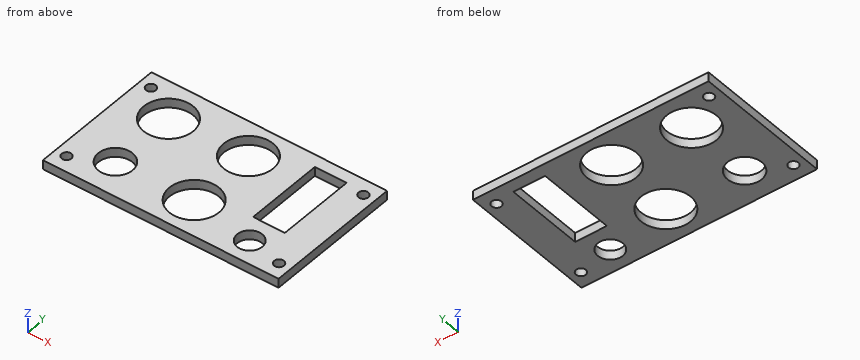
```python
from build123d import *

# Parameters (mm, degrees)
CROQUIS1_W              = 77
CROQUIS1_H              = 45
SALIENTE_EXTRUIR1_DEPTH = 3
CORTAR_EXTRUIR1_REACH   = 5
CROQUIS2_R              = 8.1
CROQUIS2_R_2            = 5.6
CROQUIS2_R_3            = 4.1
CROQUIS2_R_4            = 1.6
CROQUIS2_W              = 10.36
CROQUIS2_H              = 25.6


with BuildPart() as part:
    # Croquis1 → Saliente-Extruir1 (new body)
    with BuildSketch(Plane.XY):
        with Locations((38.5, 22.5)):
            Rectangle(CROQUIS1_W, CROQUIS1_H)
    extrude(amount=SALIENTE_EXTRUIR1_DEPTH)

    # Croquis2 → Cortar-Extruir1 (cut, up to next)
    with BuildSketch(Plane.XY.offset(3), mode=Mode.PRIVATE) as cortar_extruir1_sk1:
        with Locations((15, 33)):
            Circle(CROQUIS2_R)
    cortar_extruir1_tool1 = extrude(cortar_extruir1_sk1.sketch, amount=-CORTAR_EXTRUIR1_REACH, mode=Mode.PRIVATE) & part.part
    add(cortar_extruir1_tool1.solids().sort_by_distance((15, 33, 3))[0], mode=Mode.SUBTRACT)
    # Croquis2 → Cortar-Extruir1 (cut, up to next)
    with BuildSketch(Plane.XY.offset(3), mode=Mode.PRIVATE) as cortar_extruir1_sk2:
        with Locations((15, 11)):
            Circle(CROQUIS2_R_2)
    cortar_extruir1_tool2 = extrude(cortar_extruir1_sk2.sketch, amount=-CORTAR_EXTRUIR1_REACH, mode=Mode.PRIVATE) & part.part
    add(cortar_extruir1_tool2.solids().sort_by_distance((15, 11, 3))[0], mode=Mode.SUBTRACT)
    # Croquis2 → Cortar-Extruir1 (cut, up to next)
    with BuildSketch(Plane.XY.offset(3), mode=Mode.PRIVATE) as cortar_extruir1_sk3:
        with Locations((61.68, 7.5)):
            Circle(CROQUIS2_R_3)
    cortar_extruir1_tool3 = extrude(cortar_extruir1_sk3.sketch, amount=-CORTAR_EXTRUIR1_REACH, mode=Mode.PRIVATE) & part.part
    add(cortar_extruir1_tool3.solids().sort_by_distance((61.68, 7.5, 3))[0], mode=Mode.SUBTRACT)
    # Croquis2 → Cortar-Extruir1 (cut, up to next)
    with BuildSketch(Plane.XY.offset(3), mode=Mode.PRIVATE) as cortar_extruir1_sk4:
        with Locations((40.4, 33.95)):
            Circle(CROQUIS2_R)
    cortar_extruir1_tool4 = extrude(cortar_extruir1_sk4.sketch, amount=-CORTAR_EXTRUIR1_REACH, mode=Mode.PRIVATE) & part.part
    add(cortar_extruir1_tool4.solids().sort_by_distance((40.4, 33.95, 3))[0], mode=Mode.SUBTRACT)
    # Croquis2 → Cortar-Extruir1 (cut, up to next)
    with BuildSketch(Plane.XY.offset(3), mode=Mode.PRIVATE) as cortar_extruir1_sk5:
        with Locations((40.4, 11.45)):
            Circle(CROQUIS2_R)
    cortar_extruir1_tool5 = extrude(cortar_extruir1_sk5.sketch, amount=-CORTAR_EXTRUIR1_REACH, mode=Mode.PRIVATE) & part.part
    add(cortar_extruir1_tool5.solids().sort_by_distance((40.4, 11.45, 3))[0], mode=Mode.SUBTRACT)
    # Croquis2 → Cortar-Extruir1 (cut, up to next)
    with BuildSketch(Plane.XY.offset(3), mode=Mode.PRIVATE) as cortar_extruir1_sk6:
        with Locations((73.25, 40)):
            Circle(CROQUIS2_R_4)
    cortar_extruir1_tool6 = extrude(cortar_extruir1_sk6.sketch, amount=-CORTAR_EXTRUIR1_REACH, mode=Mode.PRIVATE) & part.part
    add(cortar_extruir1_tool6.solids().sort_by_distance((73.25, 40, 3))[0], mode=Mode.SUBTRACT)
    # Croquis2 → Cortar-Extruir1 (cut, up to next)
    with BuildSketch(Plane.XY.offset(3), mode=Mode.PRIVATE) as cortar_extruir1_sk7:
        with Locations((73.25, 5)):
            Circle(CROQUIS2_R_4)
    cortar_extruir1_tool7 = extrude(cortar_extruir1_sk7.sketch, amount=-CORTAR_EXTRUIR1_REACH, mode=Mode.PRIVATE) & part.part
    add(cortar_extruir1_tool7.solids().sort_by_distance((73.25, 5, 3))[0], mode=Mode.SUBTRACT)
    # Croquis2 → Cortar-Extruir1 (cut, up to next)
    with BuildSketch(Plane.XY.offset(3), mode=Mode.PRIVATE) as cortar_extruir1_sk8:
        with Locations((3.75, 5)):
            Circle(CROQUIS2_R_4)
    cortar_extruir1_tool8 = extrude(cortar_extruir1_sk8.sketch, amount=-CORTAR_EXTRUIR1_REACH, mode=Mode.PRIVATE) & part.part
    add(cortar_extruir1_tool8.solids().sort_by_distance((3.75, 5, 3))[0], mode=Mode.SUBTRACT)
    # Croquis2 → Cortar-Extruir1 (cut, up to next)
    with BuildSketch(Plane.XY.offset(3), mode=Mode.PRIVATE) as cortar_extruir1_sk9:
        with Locations((3.75, 40)):
            Circle(CROQUIS2_R_4)
    cortar_extruir1_tool9 = extrude(cortar_extruir1_sk9.sketch, amount=-CORTAR_EXTRUIR1_REACH, mode=Mode.PRIVATE) & part.part
    add(cortar_extruir1_tool9.solids().sort_by_distance((3.75, 40, 3))[0], mode=Mode.SUBTRACT)
    # Croquis2 → Cortar-Extruir1 (cut, up to next)
    with BuildSketch(Plane.XY.offset(3), mode=Mode.PRIVATE) as cortar_extruir1_sk10:
        with Locations((61.68, 28.3)):
            Rectangle(CROQUIS2_W, CROQUIS2_H)
    cortar_extruir1_tool10 = extrude(cortar_extruir1_sk10.sketch, amount=-CORTAR_EXTRUIR1_REACH, mode=Mode.PRIVATE) & part.part
    add(cortar_extruir1_tool10.solids().sort_by_distance((61.68, 28.3, 3))[0], mode=Mode.SUBTRACT)


solid = part.part
```
CAD build for the part. Positions are in the model's coordinates, mm. Round coordinates to 2 decimals unless told otherwise and drop trailing zeros. Order: outer loops, then holes, each group sorted by start corner. A loop starts at its lowest first (then second) coordinate and runs counter-clockwise, first axis right, second up. Notation, with made-up numbers: (-23.5, 28) -> (2.5, 28) arc R32 cw to (2.5, 62) -> close; hole circle Ø5 at (-27.75, -0.75). An arc over 180 degrees is marked (long way). Write item = value, one per line.
(1) Cut at D-D (x = 73.25). Write the cut outline in (y, z), plus the area to 3 significant figures.
Answers follow:
outline = (0, 0) -> (3.4, 0) -> (3.4, 3) -> (0, 3) -> close; (6.6, 0) -> (38.4, 0) -> (38.4, 3) -> (6.6, 3) -> close; (41.6, 0) -> (45, 0) -> (45, 3) -> (41.6, 3) -> close
area = 116 mm²
(2) Drill centre lines: L1, parallel to Y at x = 3.75, z = 1; L2, parallel to Y at x = 15, z = 1; L3, parallel to X at y = 24, z = 1.05. Where is each one in solid material? Low to high.
Answers follow:
L1 = 0 to 3.4, 6.6 to 38.4, 41.6 to 45
L2 = 0 to 5.4, 16.6 to 24.9, 41.1 to 45
L3 = 0 to 56.5, 66.86 to 77
(3) Cut at A-A (x = 15). Write the cut outline in (y, z).
Answers follow:
outline = (0, 0) -> (5.4, 0) -> (5.4, 3) -> (0, 3) -> close; (16.6, 0) -> (24.9, 0) -> (24.9, 3) -> (16.6, 3) -> close; (41.1, 0) -> (45, 0) -> (45, 3) -> (41.1, 3) -> close
(4) Cut at B-B (y = 36). Write the cut outline in (x, z).
Answers follow:
outline = (0, 0) -> (7.48, 0) -> (7.48, 3) -> (0, 3) -> close; (22.52, 0) -> (32.56, 0) -> (32.56, 3) -> (22.52, 3) -> close; (48.24, 0) -> (56.5, 0) -> (56.5, 3) -> (48.24, 3) -> close; (66.86, 0) -> (77, 0) -> (77, 3) -> (66.86, 3) -> close
(5) Cut at C-C (z = 1.05). State how many separate pieces and enclosed holes the cut face has, plus the area to 3 significant figures.
Answers follow:
separate_pieces = 1
enclosed_holes = 10
area = 2,400 mm²
